Can you work these out from the drawing? Everything is in mm from the part's minimum corner. A direction names the side the tool comes from. Coordinates: 2 decimals unless noted, no trailing zeros. Order: outer loops, then holes, each group sorted by start corner. A loop starts at its lowest first (then second) coordinate and runs counter-clockwise, first axis right, second up. Notation, with made-up numbers: (63, 7.5) -> (99, 7.5) arc R28 ccw to (99, 46.5) -> close; hole circle Ø9 at (17.5, 46). An arc over 180 degrees is marked (long way). Return JSON: item names as keys, results as strings. Group by question number.
1) For the marked faces 1, 2 and 3, which set-ups out of +Z, -Z, +X, -X, +Y, -Y let a thin tool reach every point of the face, with its end or its side?
2) If we section it at D-D, the plane x = 34.5: Please give me the cut outline in (y, z), then the cut area to 4 significant figures.
3) If we section it at A-A, the plane x = 10: Please give me the cut outline in (y, z), then the cut area to 3 significant figures.
4) If we section it at C-C, the plane y = 24.5: Please give me the cut outline in (x, z).
5) If we section it at B-B, the plane z = 11: Please give me the cut outline in (x, y), then the cut area to 3 significant figures.
6) If I drill on probe 1 along Y at (x, z) = (10, 2); probe 2 along Y at (x, z) = (30, 38); probe 3 along Z at (x, y) = (13.5, 6.75), over which ranges is the centre line in solid material (lowest first)? Write a range as from..to.
7) For pin 1 (0.9 mm diameter, centred on x = 28, z = 58.5, fed in from -Y); pin 2 (16 mm diameter, centred on x = 8.5, y = 13, fed in from +Z); pin 3 (3.5 mm diameter, centred on x = 29, y = 24, fed in from -Z); pin 4 (1 mm diameter, centred on x = 33, y = 21, fed in from +Z), each with a flat end and sliding along its axis, tell me the tip position at first contact or that it passes through.
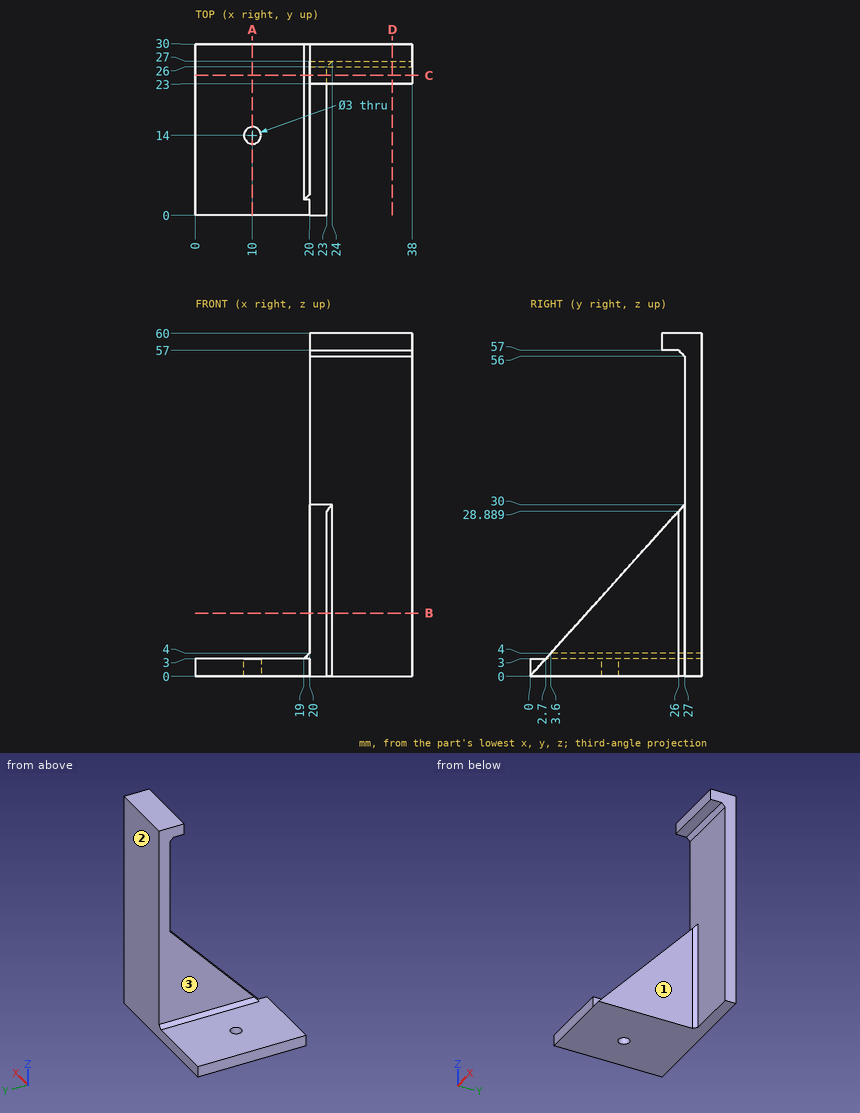
Result sheet:
{
 "1": {"face 1": "-Z, +X, -Y", "face 2": "+Z, -Z, +X, -X, +Y", "face 3": "+Z, -X, +Y, -Y"},
 "2": {"outline": "(23, 57) -> (26, 57) -> (27, 56) -> (27, 0) -> (30, 0) -> (30, 60) -> (23, 60) -> close", "area": "192.5 mm2"},
 "3": {"outline": "(0, 0) -> (12.5, 0) -> (12.5, 3) -> (0, 3) -> close; (15.5, 0) -> (30, 0) -> (30, 3) -> (15.5, 3) -> close", "area": "81.0 mm2"},
 "4": {"outline": "(0, 0) -> (23, 0) -> (23, 27.22) -> (20, 27.22) -> (20, 4) -> (19, 3) -> (0, 3) -> close; (20, 57) -> (38, 57) -> (38, 60) -> (20, 60) -> close"},
 "5": {"outline": "(20, 9.9) -> (23, 9.9) -> (23, 26) -> (24, 27) -> (38, 27) -> (38, 30) -> (20, 30) -> close", "area": "106 mm2"},
 "6": {"probe 1": "y = 0..12.5, 15.5..30", "probe 2": "y = 27..30", "probe 3": "z = 0..3"},
 "7": {"pin 1": "stops at y = 23", "pin 2": "stops at z = 3", "pin 3": "stops at z = 57", "pin 4": "passes through"}
}
